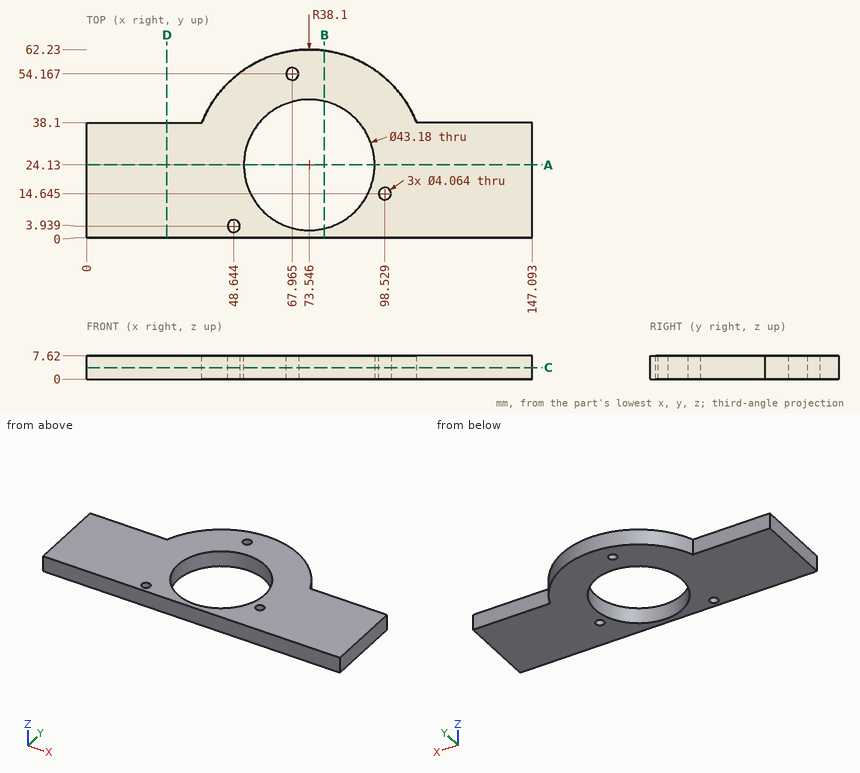
Source: three-view drawing plus pictorial views. Frame: mm from the lowest corner of the part. Coordinates: 2 decimals unless noted, no trailing zeros. Loops run counter-clockwise (first coordinate to the right, second up) from the corner with the lowest first, then second, coordinate; pieces in that order, holes last. Notation, with made-up numbers: (-20.75, 64.5) - (14.25, 64.5) arc R28 ccw to (14.25, 86.5) - close; hole circle Ø5 at (89.5, 37). An arc over 180 degrees is marked (long way). One line per item, written item: value. Start each with the question number.
1. Contact query for a flat-ended pin moving along its axis: P1, Ø2.5, axis at x = 17.5, z = 3, coming from the +Y side. Output: stop coordinate, or through.
2. Section C-C (z = 3.75). Return the cut outline in (x, y) (1 decimal).
3. Section A-A (y = 24.13). Return the cut outline in (x, z).
4. Section D-D (x = 26.5). Return the cut outline in (y, z), and give its area (3 significant figures).
5. Section B-B (x = 78.5). Return the cut outline in (y, z).
6. Ray query, L1, parallel to X at y = 23, z = 6.75; L2, parallel to Y at x = 121, z = 3.5; L3, parallel to Y at x = 59.5, z = 7 (1 decimal). Return the intervals inside material, ascending.
Verdict:
1. P1: stops at y = 38.1
2. outline: (0, 0) - (147.1, 0) - (147.1, 38.1) - (109, 38.1) arc R38.1 ccw to (38.1, 38.1) - (0, 38.1) - close; hole circle Ø4.1 at (48.6, 3.9); hole circle Ø43.2 at (73.5, 24.1); hole circle Ø4.1 at (68, 54.2); hole circle Ø4.1 at (98.5, 14.6)
3. outline: (0, 0) - (51.96, 0) - (51.96, 7.62) - (0, 7.62) - close; (95.14, 0) - (147.09, 0) - (147.09, 7.62) - (95.14, 7.62) - close
4. outline: (0, 0) - (38.1, 0) - (38.1, 7.62) - (0, 7.62) - close
4. area: 290 mm2
5. outline: (0, 0) - (3.12, 0) - (3.12, 7.62) - (0, 7.62) - close; (45.14, 0) - (61.91, 0) - (61.91, 7.62) - (45.14, 7.62) - close
6. L1: x = 0 to 51.99, 95.11 to 147.09
6. L2: y = 0 to 38.1
6. L3: y = 0 to 7.7, 40.5 to 59.5
